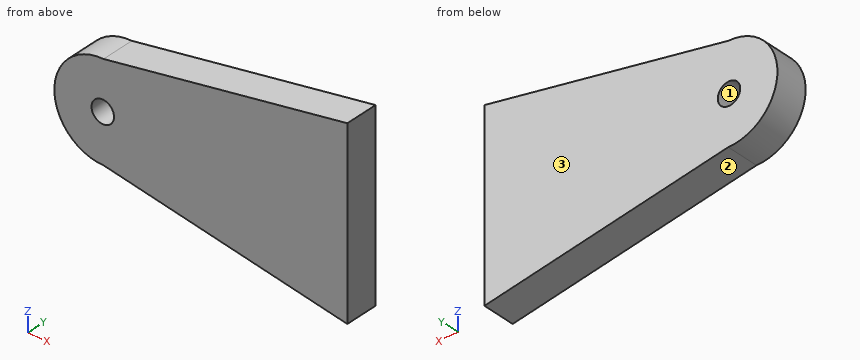
Autodesk Inventor part; units mm, degrees
ref_plane "YZ Plane" through (0, 0, 0) normal (1, 0, 0) x (0, 1, 0)
ref_plane "XZ Plane" through (0, 0, 0) normal (0, 1, 0) x (-1, 0, 0)
ref_plane "XY Plane" through (0, 0, 0) normal (0, 0, 1) x (1, 0, 0)
sketch "Sketch1" plane through (0, 0, 0) normal (0, 1, 0) x (-1, 0, 0)
  line L0 (0, 0) -> (0, -30)
  line L1 (0, 0) -> (39.9996, -7.053)
  line L2 (0, -30) -> (39.9998, -22.947)
  arc A0 (39.9998, -22.947) -> (39.9996, -7.053) centre (40.1288, -15) ccw
  dimension "d0" = 30
  dimension "d1" = 80
  dimension "d4" = 80
  dimension "d7" = 15.896
  dimension "d9" = 40.1288
  dimension "d10" = 7.8038
extrude "Extrusion1" add sketch "Sketch1" along normal blind 5.5
hole "Hole1" at (-40.1288, 0, -15) direction (0, 1, 0) diameter 3.6881 depth 13 tip angle 118
properties part number "wea abajo movil"
Source: CAD feature listing. Evaluate the final solid. Frame: model axes, mm. Face numbers are marked on the shaded views. Give positions to 0.01 mm unless a question says otherwise; leave off trailing zeros. Write each loop counter-clockwise with the first axis right and the second up, starting at its lowest first coordinate (ties: lowest second). Pieces come first, ordered by that corner, then holes.
1. Section query C-C (x = -17). Return the cut outline in (y, z), then the cut area to 3 significant figures.
2. Section query A-A (z = -15). Return the cut outline in (x, y), then the cut area to 3 significant figures.
3. Section query B-B (y = 3.8). Return the cut outline in (x, z), then the cut area to 3 significant figures.
4. Material intervals for line 1 along X through (y, z) = (3.55, -15); line 2 along Z through (x, y) = (-38.5, 4.5); line 3 along X through (y, z) = (3.25, -22), sorted ascending.
5. Section query D-D (z = -6.5). Return the cut outline in (x, y).
6. Pull-direction query (X, two-part tool) for the marked faces 1, 2 and 3; classes: +X half, -X half, draft (parallel to the pull), parting line (faces both ways), or undercut.
7. First-contact query: pin 1 (3 mm diameter, centred on x = -40.13, z = -15, fed in from -Y); pin 2 (3 mm diameter, centred on y = 2.5, z = -19.5, fed in from -X); pin 3 (1.5 mm diameter, centred on x = -41.5, y = 3.5, fed in from +Z); pin 4 (1 mm diameter, centred on y = 1.5, z = -11, fed in from -X). Flat tips, straight axial feed; report the tip coordinate or a pass-through.
Output values:
1. outline: (0, -27) - (5.5, -27) - (5.5, -3) - (0, -3) - close
1. area: 132 mm2
2. outline: (-48.08, 0) - (-41.97, 0) - (-41.97, 5.5) - (-48.08, 5.5) - close; (-38.28, 0) - (0, 0) - (0, 5.5) - (-38.28, 5.5) - close
2. area: 244 mm2
3. outline: (-40, -22.95) - (0, -30) - (0, 0) - (-40, -7.05) arc R7.95 ccw (long way) to start; hole circle Ø3.69 at (-40.13, -15)
3. area: 1,010 mm2
4. line 1: x = -48.08 to -41.97, -38.28 to 0
4. line 2: z = -23.21 to -15.86, -14.14 to -6.79
4. line 3: x = -43.89 to 0
5. outline: (-36.86, 0) - (0, 0) - (0, 5.5) - (-36.86, 5.5) - close
6. face 1: undercut
6. face 2: -X half
6. face 3: draft
7. pin 1: passes through
7. pin 2: stops at x = -47.49
7. pin 3: stops at z = -7.08
7. pin 4: stops at x = -47.26
